For this review, use the dimensioned drawing (mm, ordinates from the lowest corner) and the shaded views. Round coordinates to 2 decimals unless told otherwise and drop trailing zeros. Order: outer loops, then holes, each group sorted by start corner. A loop starts at its lowest first (then second) coordinate and runs counter-clockwise, first axis right, second up. Notation, with made-up numbers: M 22,-23 L 26,-23 A10 cw 26,-8 Z; hole C -31.5,38.25 d11. An arc over 180 degrees is marked long. Use a Markdown table: item, result. Add a question column.
1. Insertion check: P1, Ø0.6, axis at x = 12.5, y = 0, coming from the +Z side; P2, Ø2, axis at x = 13.5, z = 3, coming from the -Y side. Each pin has a flat end and moves straight along its axis. Give the tip position at first contact, or say it passes through.
2. Consider section B-B on z = 7.75. State the section outline as (x, y) points, then the cut area to 3 significant figures.
3. The part is to be moulded in two halves that separate along Z. For the marked faces 1 and 2, say which applies: +Z half, -Z half, draft (parallel to the pull), parting line (faces both ways), or undercut.
4. Consider section D-D on z = 13. State the section outline as (x, y) points.
5. To check wall thickness, follow probe 1 along X at (y, z) = (1.5, 7.25); probe 2 along X at (y, z) = (0.3, 6); probe 3 along Z at (x, y) = (16.5, 0.25) (1 decimal). State the ranges of each line that lie inside material, in increasing order.
6. Consider section A-A on x = 10. State the section outline as (y, z) points (1 decimal).
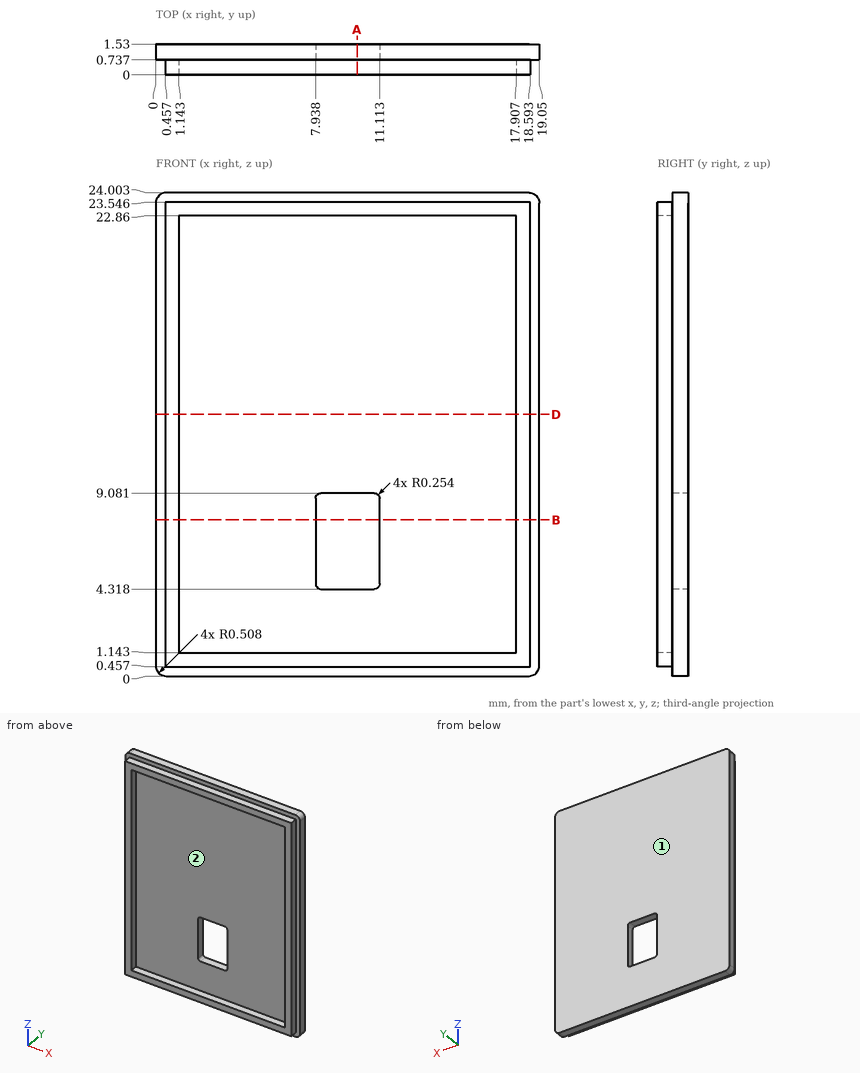
Answer block:
| question | item | result |
|---|---|---|
| 1 | P1 | z = 23.55 |
| 1 | P2 | y = 0.74 |
| 2 | outline | M 0,0.74 L 0.46,0.74 L 0.46,0 L 1.14,0 L 1.14,0.74 L 7.94,0.74 L 7.94,1.53 L 0,1.53 Z; M 11.11,0.74 L 17.91,0.74 L 17.91,0 L 18.59,0 L 18.59,0.74 L 19.05,0.74 L 19.05,1.53 L 11.11,1.53 Z |
| 2 | area | 13.6 mm^2 |
| 3 | face 1 | draft |
| 3 | face 2 | undercut |
| 4 | outline | M 0,0.74 L 0.46,0.74 L 0.46,0 L 1.14,0 L 1.14,0.74 L 17.91,0.74 L 17.91,0 L 18.59,0 L 18.59,0.74 L 19.05,0.74 L 19.05,1.53 L 0,1.53 Z |
| 5 | probe 1 | 0 to 7.94, 11.11 to 19.05 |
| 5 | probe 2 | 0.46 to 1.14, 17.91 to 18.59 |
| 5 | probe 3 | 0.5 to 1.1, 22.9 to 23.5 |
| 6 | outline | M 0,0.5 L 0.7,0.5 L 0.7,0 L 1.5,0 L 1.5,4.3 L 0.7,4.3 L 0.7,1.1 L 0,1.1 Z; M 0,22.9 L 0.7,22.9 L 0.7,9.1 L 1.5,9.1 L 1.5,24 L 0.7,24 L 0.7,23.5 L 0,23.5 Z |
